Check sheet for the drawn part. Datum: minimum x, y, z corner. Units: mm. Coordinates: 2 decimals unless noted, no trailing zeros. Write each loop counter-clockwise with the first axis right and the second up, starting at its lowest first coordinate (ties: lowest second). Pieces come first, ordered by that corner, then holes. Notation, with made-up numbers: (2.5, 87) - (24.5, 87) arc R19 cw to (24.5, 112) - close; hole circle Ø9 at (83.5, 10.5). An arc over 180 degrees is marked (long way). Use CSV: the item, a comma, the result in double quotes. Start each with the question number.
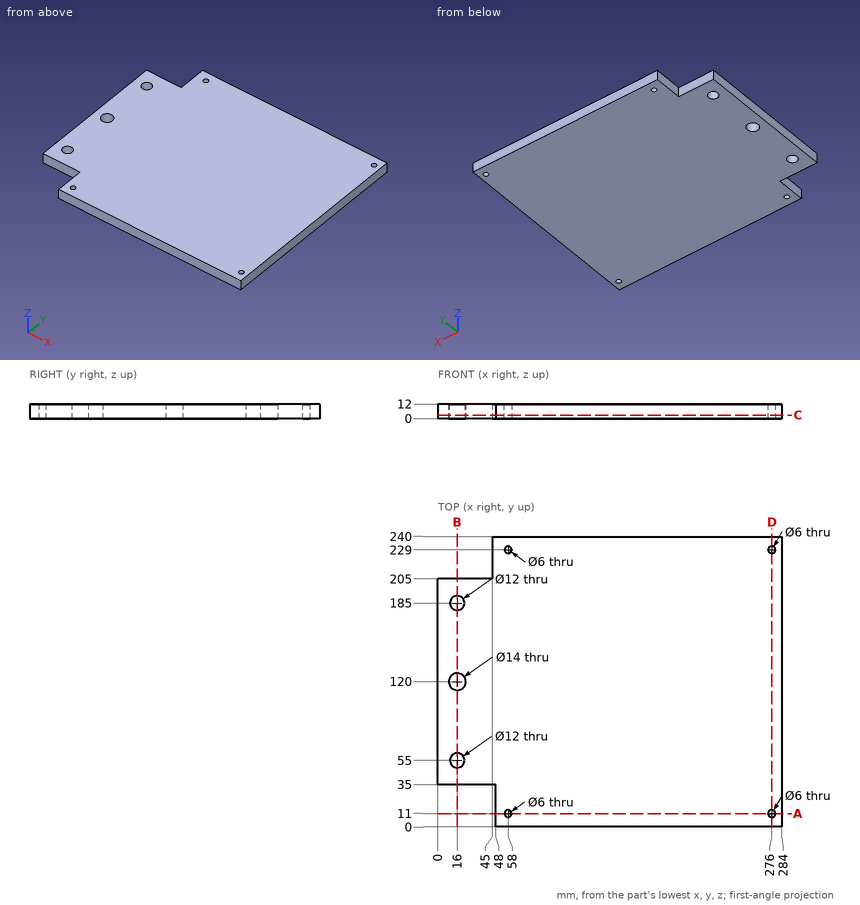
Q1. Cross-section at C-C (z = 2.75). Record the cut outline in (x, y).
Q2. Gauge pin test, flat ends, axial feed: pin 1 (6 mm diameter, centred on y = 223, z = 9, fed in from -X); pin 2 (6 mm diameter, centred on x = 26.5, z = 6.5, fed in from +Y); pin 3 (6 mm diameter, centred on x = 23, z = 7, fed in from -Y). Record the tip position at first contact, or that the pin passes through.
Q3. Cross-section at A-A (y = 11). Record the cut outline in (x, z).
Q4. Cross-section at D-D (x = 276). Record the cut outline in (y, z), plus the area to 3 significant figures.
Q5. Cross-section at B-B (x = 16). Record the cut outline in (y, z).
Q6. Scan lines: line 1 along Y through (x, z) = (16, 6.5); line 2 along X through (y, z) = (229, 3.25); line 3 along Y through (x, z) = (58, 3.5). Record each from-to range of solid material in increasing order. Write a range as from..to.
Reply:
1,outline,"(0, 35) - (48, 35) - (48, 0) - (284, 0) - (284, 240) - (45, 240) - (45, 205) - (0, 205) - close; hole circle Ø14 at (16, 120); hole circle Ø12 at (16, 55); hole circle Ø12 at (16, 185); hole circle Ø6 at (58, 11); hole circle Ø6 at (58, 229); hole circle Ø6 at (276, 11); hole circle Ø6 at (276, 229)"
2,pin 1,"x = 45"
2,pin 2,"y = 205"
2,pin 3,"y = 35"
3,outline,"(48, 0) - (55, 0) - (55, 12) - (48, 12) - close; (61, 0) - (273, 0) - (273, 12) - (61, 12) - close; (279, 0) - (284, 0) - (284, 12) - (279, 12) - close"
4,outline,"(0, 0) - (8, 0) - (8, 12) - (0, 12) - close; (14, 0) - (226, 0) - (226, 12) - (14, 12) - close; (232, 0) - (240, 0) - (240, 12) - (232, 12) - close"
4,area,"2,740 mm^2"
5,outline,"(35, 0) - (49, 0) - (49, 12) - (35, 12) - close; (61, 0) - (113, 0) - (113, 12) - (61, 12) - close; (127, 0) - (179, 0) - (179, 12) - (127, 12) - close; (191, 0) - (205, 0) - (205, 12) - (191, 12) - close"
6,line 1,"35..49, 61..113, 127..179, 191..205"
6,line 2,"45..55, 61..273, 279..284"
6,line 3,"0..8, 14..226, 232..240"
